Answer from the drawing. Dimensions are ordinates in mm from the lowest x, y and z of the part. A direction names the side the tool comes from. Round coordinates to 2 decimals unless told otherwise and drop trailing zeros. Write each loop counter-clockwise with the first axis right and the second up, starting at its lowest first coordinate (ties: lowest second). Pieces come first, ordered by that corner, then holes. Notation, with made-up numbers: M 71.25,-30.5 L 113.25,-30.5 A27 ccw 113.25,-1.5 Z; hole C 79,36 d6. An arc over 180 degrees is marked long. One line per item, written item: value. Start each with the question number.
(1) Section B-B (y = 16.5) is taken. Determine the outline of the cut face in (x, z).
(2) Consider probe 1 along X at (y, z) = (81.2, 5.4); probe 2 along Y at (x, z) = (25.5, 5.35); probe 3 along Y at (x, z) = (25.5, 6.9). Determine where each line is inside the solid, lowest interval first.
(3) Section A-A (y = 81.2) is taken. Determine the outline of the cut face in (x, z).
(4) Given P1, Ø4, axis at x = 25.5, y = 81.2, coming from the +Z side; P2, Ø10, axis at x = 27, y = 82, coming from the -Z side; P3, Ø5.5, axis at y = 59.5, z = 2, coming from the +X side, each flat-ended and moving along its own axis, determine where each tip first touches the part or whether it passes through.
(5) Section C-C (x = 35) is taken. Determine the outline of the cut face in (y, z).
(6) For the marked faces 1 and 2, determine the directions among +Z, -Z, +X, -X, +Y, -Y from which every point of the face is accessible in a straight line to the end or side of a thin tool.
(7) Section D-D (z = 1.5) is taken. Determine the outline of the cut face in (x, y), plus the area to 3 significant figures.
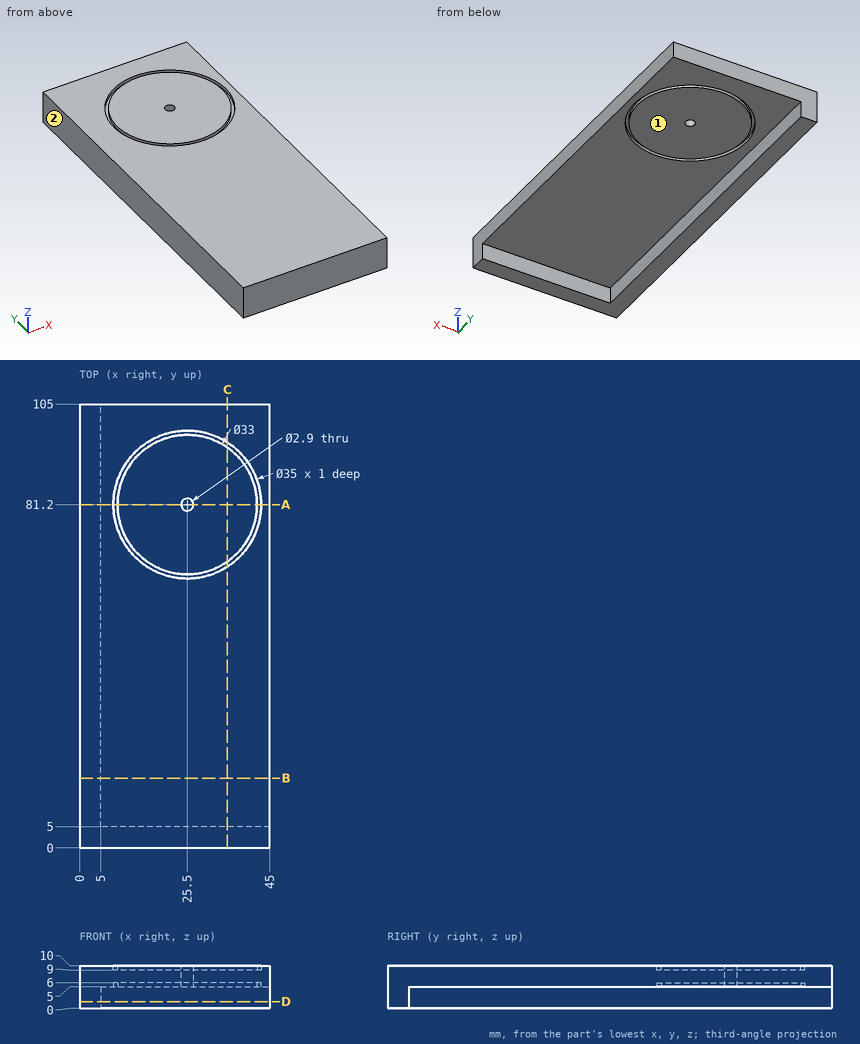
Recorded:
1. outline: M 0,0 L 5,0 L 5,5 L 45,5 L 45,10 L 0,10 Z
2. probe 1: x = 0 to 8, 9 to 24.05, 26.95 to 42, 43 to 45
2. probe 2: y = 0 to 63.7, 64.7 to 79.75, 82.65 to 97.7, 98.7 to 105
2. probe 3: y = 0 to 79.75, 82.65 to 105
3. outline: M 0,0 L 5,0 L 5,5 L 8,5 L 8,6 L 9,6 L 9,5 L 24.05,5 L 24.05,10 L 9,10 L 9,9 L 8,9 L 8,10 L 0,10 Z; M 26.95,5 L 42,5 L 42,6 L 43,6 L 43,5 L 45,5 L 45,10 L 43,10 L 43,9 L 42,9 L 42,10 L 26.95,10 Z
4. P1: stops at z = 10
4. P2: stops at z = 5
4. P3: stops at x = 5
5. outline: M 0,0 L 5,0 L 5,5 L 66.5,5 L 66.5,6 L 67.71,6 L 67.71,5 L 94.69,5 L 94.69,6 L 95.9,6 L 95.9,5 L 105,5 L 105,10 L 95.9,10 L 95.9,9 L 94.69,9 L 94.69,10 L 67.71,10 L 67.71,9 L 66.5,9 L 66.5,10 L 0,10 Z
6. face 1: -Z, +X, +Y
6. face 2: +Z, -Z, -X, +Y, -Y
7. outline: M 0,0 L 45,0 L 45,5 L 5,5 L 5,105 L 0,105 Z
7. area: 725 mm2
